from build123d import *

# Parameters (mm, degrees)
SKETCH1_W           = 406.4
SKETCH1_H           = 127
BOSS_EXTRUDE1_DEPTH = 5.715
SKETCH2_W           = 50.8
SKETCH2_H           = 5.715
TOP_JIGSAW_DEPTH    = 6.715
SKETCH3_W           = 5.715
SKETCH3_H           = 25.4
RIGHT_JIGSAW_DEPTH  = 6.715
SKETCH4_W           = 0.254
SKETCH4_H           = 5.715
SKETCH4_W_2         = 5.715
SKETCH4_H_2         = 0.254
BOSS_EXTRUDE2_DEPTH = 5.715


with BuildPart() as part:
    # Sketch1 → Boss-Extrude1 (new body)
    with BuildSketch(Plane.XY):
        Rectangle(SKETCH1_W, SKETCH1_H)
    extrude(amount=BOSS_EXTRUDE1_DEPTH)

    # Sketch2 → Top Jigsaw (cut, through all)
    with BuildSketch(Plane.XY.offset(5.715)):
        with Locations((-152.4, 60.6425)):
            Rectangle(SKETCH2_W, SKETCH2_H)
        with Locations((-76.2, 60.6425)):
            Rectangle(SKETCH2_W, SKETCH2_H)
        with Locations((0, 60.6425)):
            Rectangle(SKETCH2_W, SKETCH2_H)
        with Locations((76.2, 60.6425)):
            Rectangle(SKETCH2_W, SKETCH2_H)
        with Locations((152.4, 60.6425)):
            Rectangle(SKETCH2_W, SKETCH2_H)
    top_jigsaw = extrude(amount=-TOP_JIGSAW_DEPTH, mode=Mode.SUBTRACT)

    # Bottom Jigsaw: Top Jigsaw across plane
    add(top_jigsaw.mirror(Plane.ZX), mode=Mode.SUBTRACT)

    # Sketch3 → Right Jigsaw (cut, through all)
    with BuildSketch(Plane.XY.offset(5.715)):
        with Locations((200.3425, 25.4)):
            Rectangle(SKETCH3_W, SKETCH3_H)
        with Locations((200.3425, -25.4)):
            Rectangle(SKETCH3_W, SKETCH3_H)
    right_jigsaw = extrude(amount=-RIGHT_JIGSAW_DEPTH, mode=Mode.SUBTRACT)

    # Mirror2: Right Jigsaw across plane
    add(right_jigsaw.mirror(Plane(origin=(0, 0, 0), x_dir=(0, 0, 1), z_dir=(1, 0, 0))), mode=Mode.SUBTRACT)

    # Sketch4 → Boss-Extrude2 (add)
    with BuildSketch(Plane.XY.offset(5.715)):
        with Locations((-177.673, 60.6425)):
            Rectangle(SKETCH4_W, SKETCH4_H)
        with Locations((-127.127, 60.6425)):
            Rectangle(SKETCH4_W, SKETCH4_H)
        with Locations((-101.473, 60.6425)):
            Rectangle(SKETCH4_W, SKETCH4_H)
        with Locations((-50.927, 60.6425)):
            Rectangle(SKETCH4_W, SKETCH4_H)
        with Locations((-25.273, 60.6425)):
            Rectangle(SKETCH4_W, SKETCH4_H)
        with Locations((25.273, 60.6425)):
            Rectangle(SKETCH4_W, SKETCH4_H)
        with Locations((50.927, 60.6425)):
            Rectangle(SKETCH4_W, SKETCH4_H)
        with Locations((101.473, 60.6425)):
            Rectangle(SKETCH4_W, SKETCH4_H)
        with Locations((127.127, 60.6425)):
            Rectangle(SKETCH4_W, SKETCH4_H)
        with Locations((177.673, 60.6425)):
            Rectangle(SKETCH4_W, SKETCH4_H)
        with Locations((200.3425, 37.973)):
            Rectangle(SKETCH4_W_2, SKETCH4_H_2)
        with Locations((200.3425, 12.827)):
            Rectangle(SKETCH4_W_2, SKETCH4_H_2)
        with Locations((-200.3425, 37.973)):
            Rectangle(SKETCH4_W_2, SKETCH4_H_2)
        with Locations((-200.3425, 12.827)):
            Rectangle(SKETCH4_W_2, SKETCH4_H_2)
    boss_extrude2 = extrude(amount=-BOSS_EXTRUDE2_DEPTH)

    # Mirror3: Boss-Extrude2 across plane
    add(boss_extrude2.mirror(Plane.ZX))


solid = part.part
The listing builds one solid part. Answer for the finished solid, in the listing's coordinates (mm). Coordinates: 2 decimals unless noted, no trailing zeros. Order: outer loops, then holes, each group sorted by start corner. A loop starts at its lowest first (then second) coordinate and runs counter-clockwise, first axis right, second up. Notation, with made-up numbers: (21, 86) -> (51, 86) arc R26 cw to (51, 106) -> close; hole circle Ø10 at (-9.75, 33). An arc over 180 degrees is marked (long way). Answer in a Markdown table with one row per item. Add a question column.
Item 1: Each of these flat-tipped pins is pushed along its axis until it touches: P1, Ø3, axis at y = -30, z = 2.5, coming from the -X side (3 decimals); P2, Ø1.5, axis at y = -14, z = 1, coming from the +X side (3 decimals). Where does it stop, or does it pass through?
Item 2: Find section B-B (y = 24). Write down the section's boundary in (x, z) (3 decimals), then the cut area to 3 significant figures.
Item 3: Find the intervals of material crossed by L1, parallel to X at y = 28, z = 1.75 (3 decimals); L2, parallel to Y at x = -154, z = 1.85 (3 decimals), in increasing order. Write a range as from..to.
Item 4: Determine the mould class of faces 1 (the face through (-3, -1, 0)), 2 (the face through (-3, -1, 5.715)) for opening direction Z: +Z half, -Z half, draft (parallel to the pull), parting line (faces both ways), or undercut.
Item 5: Find section A-A (x = -73). Write down the section's boundary in (y, z) (3 decimals), then the cut area to 3 significant figures.
Result set:
| question | item | result |
|---|---|---|
| 1 | P1 | stops at x = -197.485 |
| 1 | P2 | stops at x = 197.485 |
| 2 | outline | (-197.485, 0) -> (197.485, 0) -> (197.485, 5.715) -> (-197.485, 5.715) -> close |
| 2 | area | 2,260 mm² |
| 3 | L1 | x = -197.485..197.485 |
| 3 | L2 | y = -57.785..57.785 |
| 4 | face 1 | -Z half |
| 4 | face 2 | +Z half |
| 5 | outline | (-57.785, 0) -> (57.785, 0) -> (57.785, 5.715) -> (-57.785, 5.715) -> close |
| 5 | area | 660 mm² |
